Check sheet for the modelled part. Datum: model origin and axes. Units: mm. A direction names the side the tool comes from. Round coordinates to 2 decimals unless told otherwise and drop trailing zeros. Order: outer loops, then holes, each group sorted by start corner. A loop starts at its lowest first (then second) coordinate and runs counter-clockwise, first axis right, second up.
(1) Mould release check, pull along X, two halves, no side actions. Record for faces 1 (the flat face through (0, -72, 7)), 2 (the flat face through (17.5, 10, 5)), 3 (the cylindrical face through (19.408, -0.651, 10.103)): released by +X, released by -X, zero draft, split by the parting line, or undercut.
(2) Sectioned sample at A-A, the plane x = 0. Enter the section's corners in (y, z), and give its area (4 significant figures).
(3) Sectioned sample at B-B, the plane z = 0. Enter the section's corners in (x, y), and give its area (3 significant figures).
(4) Sectioned sample at C-C, the plane z = 18.5. Enter the section's corners in (x, y), and give its area (3 significant figures).
(5) Depth check by flat-ended pin: pin 1 (3 mm diameter, centred on y = 13.5, z = 8, fed in from -X); pin 2 (6 mm diameter, centred on y = -5.5, z = -4, fed in from +X); pin 3 (1.2 mm diameter, centred on x = -17, y = 0, fed in from +Z). Enter the tip coordinate at first touch or a pass-through.
(6) Sectioned sample at D-D, the plane y = -26.5. Enter the section's corners in (x, z).
(7) Thickness scan on probe 1 along X at (y, z) = (12.5, 0.5); probe 2 along X at (y, z) = (-61, 10.5); probe 3 along Y at (x, z) = (-29, 14). Record the ranges inside material, lowest first.
(8) Tool access check on faces 4 (the flat face through (0, -34, -5)), 5 (the flat face through (-17.5, 10, 5)), 6 (the flat face through (-8.6, 14, 5)). Record the directions out of +Z, -Z, +X, -X, +Y, -Y that give a thin tool (end or side, any length) a straight path to the whole face; none if there is none.
Autodesk Fusion 360 part; units mm, degrees
sketch "草图1" plane through (0, 0, 0) normal (0, 0, 1) x (1, 0, 0)
  line L0 (-8.6, 11.0472) -> (-8.6, 16.9)
  line L1 (8.6, 11.0472) -> (8.6, 16.9)
  arc A0 (-8.6, 11.0472) -> (8.6, 11.0472) centre (0, 0) ccw
  line L2 (-17.5, 16.9) -> (-8.6, 16.9)
  line L3 (8.6, 16.9) -> (17.5, 16.9)
  line L4 (0, -14) -> (0, 27.4039)
  circle A1 centre (-17.2022, 0.6702) radius 2
  circle A2 centre (17.5, -0.05) radius 2
  line L5 (17.5, 16.9) -> (17.5, 1.95)
  line L6 (17.5, -2.05) -> (17.5, -17)
  line L7 (-17.5, -17) -> (-17.5, -1.3076)
  line L8 (-17.5, 2.6479) -> (-17.5, 16.9)
  line L9 (17.5, -17) -> (17.5, -67)
  line L10 (17.5, -67) -> (-17.5, -67)
  line L11 (-17.5, -67) -> (-17.5, -17)
  line L12 (35, -72) -> (-35, -72)
  line L13 (-35, -72) -> (-35, -67)
  line L14 (35, -67) -> (35, -72)
  line L15 (-35, -67) -> (35, -67)
  dimension "d1" = 28
  dimension "d6" = 17.2
  dimension "d9" = 4
  dimension "d10" = 4
  dimension "d15" = 50
extrude "拉伸3" add sketch "草图1" along normal blind 15 contours L0 L1 A0 L2 L3 A1 A2 L5 L6 L7 L8 L9 L10 L11 L15
extrude "拉伸4" add sketch "草图1" along normal blind 20 contours A1 | A2
extrude "拉伸5" add sketch "草图1" against normal blind 5 contours L0 L1 A0 L2 L3 A1 A2 L5 L6 L7 L8 L9 L10 L11 L15
extrude "拉伸6" add sketch "草图1" against normal blind 5 contours A1 | A2
extrude "拉伸7" add sketch "草图1" along normal blind 20 contours L10 L12 L13 L14 L15
extrude "拉伸8" add sketch "草图1" against normal blind 10 contours L10 L12 L13 L14 L15
extrude "拉伸9" add 1 faces at (-11.6667, -68.6667, 20) along direction (0, 0, 1) blind 5
Derived:
1. face 1: zero draft
1. face 2: released by +X
1. face 3: undercut
2. outline: (-72, -10) - (-67, -10) - (-67, -5) - (-14, -5) - (-14, 15) - (-67, 15) - (-67, 25) - (-72, 25) - close
2. area: 1,235 mm2
3. outline: (-35, -72) - (35, -72) - (35, -67) - (17.5, -67) - (17.5, -2.05) arc R2 ccw to (17.5, 1.95) - (17.5, 16.9) - (8.6, 16.9) - (8.6, 11.05) arc R14 cw (long way) to (-8.6, 11.05) - (-8.6, 16.9) - (-17.5, 16.9) - (-17.5, 2.65) arc R2 ccw to (-17.5, -1.31) - (-17.5, -67) - (-35, -67) - close
3. area: 2,620 mm2
4. outline: (-35, -72) - (35, -72) - (35, -67) - (-35, -67) - close; circle Ø4 at (-17.2, 0.67); circle Ø4 at (17.5, -0.05)
4. area: 375 mm2
5. pin 1: stops at x = -17.5
5. pin 2: stops at x = 17.5
5. pin 3: stops at z = 20
6. outline: (-17.5, -5) - (17.5, -5) - (17.5, 15) - (-17.5, 15) - close
7. probe 1: x = -17.5 to -8.6, 8.6 to 17.5
7. probe 2: x = -17.5 to 17.5
7. probe 3: y = -72 to -67
8. face 4: -Z, +X, -X, +Y
8. face 5: +Z, -Z, -X, +Y
8. face 6: +Z, -Z, +Y
